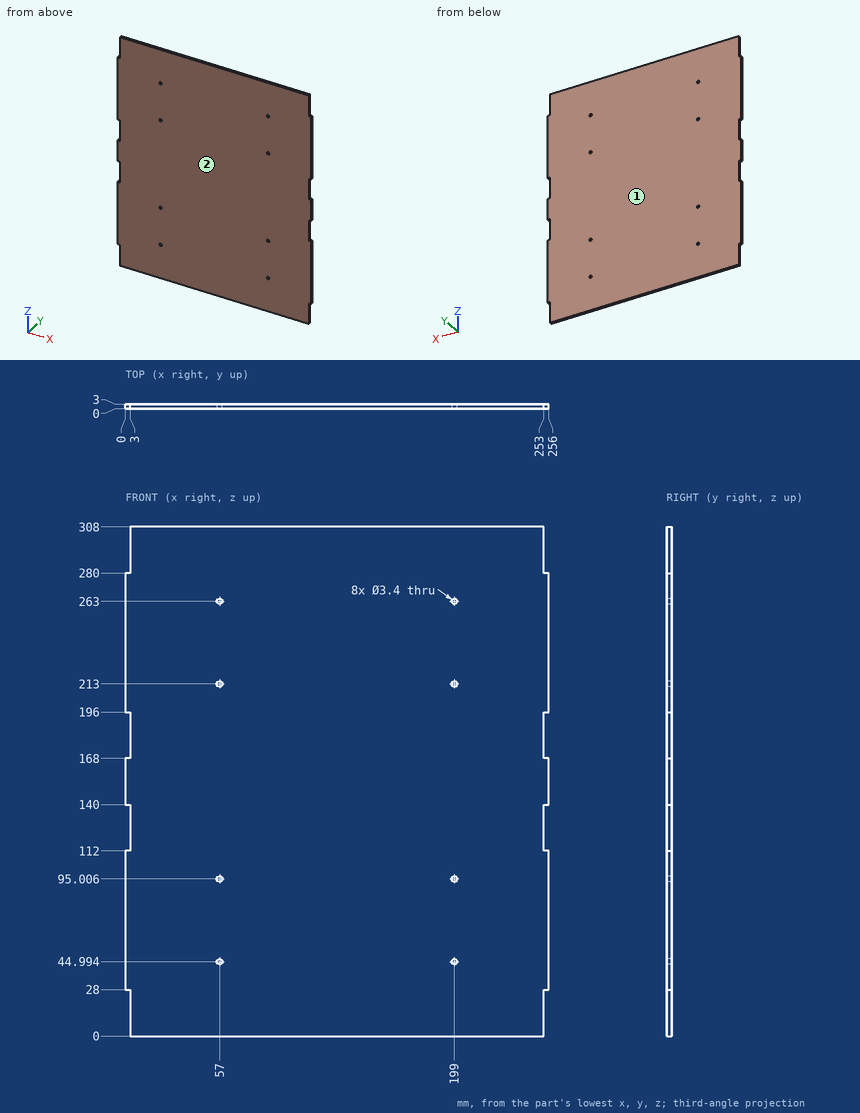
Source: three-view drawing plus pictorial views. Frame: mm from the lowest corner of the part. Round coordinates to 2 decimals unless told otherwise and drop trailing zeros. Answer as CSV lines item,"result". Start each with the question number.
(1) Line query: line 1 (Z direction, x = 57, y = 0.65); line 2 (X direction, y = 1, z = 213); line 3 (X direction, y = 1.7, z = 127). Output: solid intervals per line, ascending. Write a range as [from, to].
(2) Draft query along Y for the marked faces 1 and 2. Return one class per face: released by +Y, released by -Y, zero draft, split by the parting line, or undercut.
(3) First-contact query: pin 1 (0.9 mm diameter, centred on y = 1, z = 19.5, fed in from -X); pin 2 (0.9 mm diameter, centred on y = 1.5, z = 7, fed in from +X); pin 3 (1.5 mm diameter, centred on x = 254.5, y = 1, fed in from +Z). Flat tips, straight axial feed; report the tip coordinate or a pass-through.
Values found:
1,line 1,"z = [0, 43.29], [46.69, 93.31], [96.71, 211.3], [214.7, 261.3], [264.7, 308]"
1,line 2,"x = [0, 55.3], [58.7, 197.3], [200.7, 256]"
1,line 3,"x = [3, 253]"
2,face 1,"released by +Y"
2,face 2,"released by -Y"
3,pin 1,"stops at x = 3"
3,pin 2,"stops at x = 253"
3,pin 3,"stops at z = 280"
